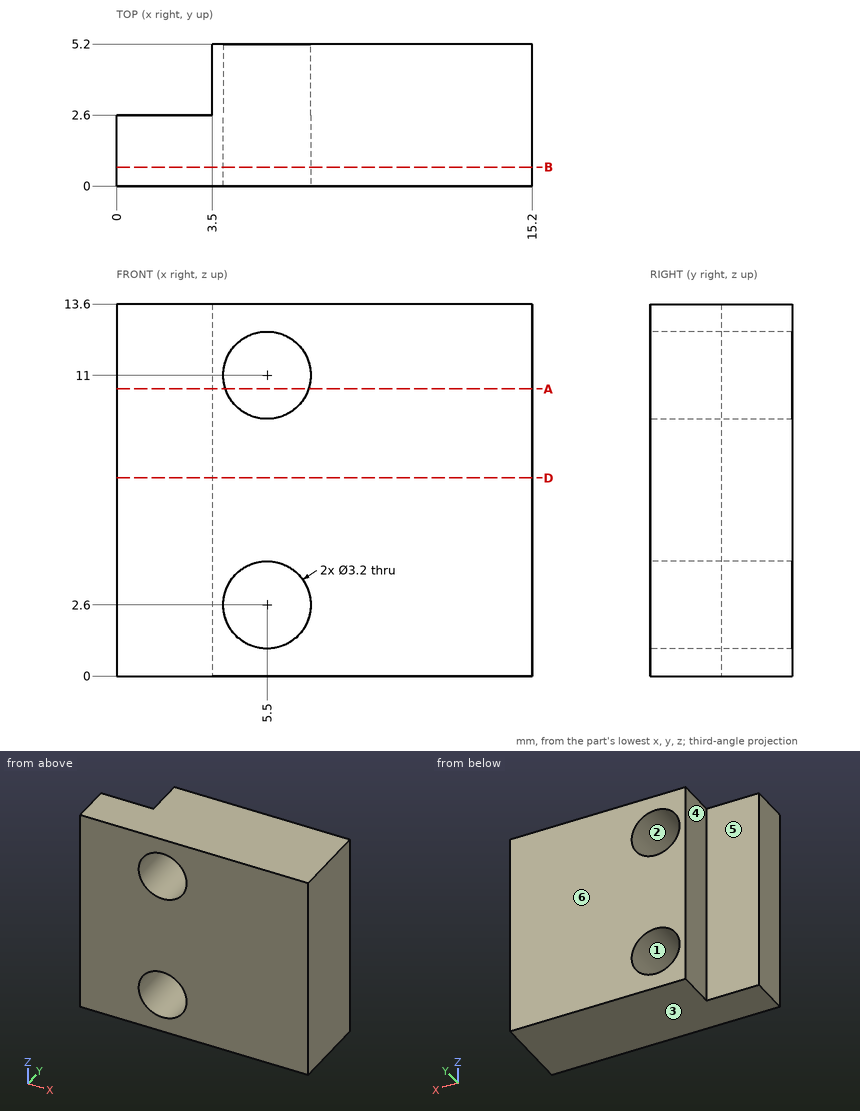
For this review, use the dimensioned drawing (mm, ordinates from the lowest corner) and the shaded views. A direction names the side the tool comes from. Round coordinates to 2 decimals unless told otherwise and drop trailing zeros. Write each loop counter-clockwise with the first axis right and the second up, starting at its lowest first coordinate (ties: lowest second). Pieces come first, ordered by that corner, then holes. Notation, with made-up numbers: (34, 69) - (76, 69) arc R17 cw to (76, 76) - close; hole circle Ø9 at (61, 28). An arc over 180 degrees is marked (long way). Answer as a JSON object with one key per item and string values.
1. Tool access review of the marked faces 5 and 6: name each direction out of +Z, -Z, +X, -X, +Y, -Y from which nothing blocks a thin tool from reaching the whole face with its end or side.
Response values:
{"face 5": "+Z, -Z, -X, +Y", "face 6": "+Z, -Z, +X, -X, +Y"}
2. We need section A-A on z = 10.5. Give the boundary of the cut face in (x, y).
Response values:
{"outline": "(0, 0) - (3.98, 0) - (3.98, 5.2) - (3.5, 5.2) - (3.5, 2.6) - (0, 2.6) - close; (7.02, 0) - (15.2, 0) - (15.2, 5.2) - (7.02, 5.2) - close"}
3. We need section D-D on z = 7.25. Give the boundary of the cut face in (x, y).
Response values:
{"outline": "(0, 0) - (15.2, 0) - (15.2, 5.2) - (3.5, 5.2) - (3.5, 2.6) - (0, 2.6) - close"}
4. For pin 1 Ø3 at (x, z) = (5.5, 11) entering from -Y; pin 2 Ø2 at (y, z) = (4, 8) entering from -X; pin 3 Ø1 at (x, z) = (2, 7) entering from +Y, all flat-tipped, find the tip position at first contact; note any pin that passes through.
Response values:
{"pin 1": "passes through", "pin 2": "stops at x = 3.5", "pin 3": "stops at y = 2.6"}
5. To check wall thickness, follow line 1 along Z through (x, y) = (5.5, 1.3); line 2 along X through (y, z) = (1.7, 2.6); line 3 along X through (y, z) = (2.8, 11). State the ranges of each line that lie inside material, in increasing order.
Response values:
{"line 1": "z = 0 to 1, 4.2 to 9.4, 12.6 to 13.6", "line 2": "x = 0 to 3.9, 7.1 to 15.2", "line 3": "x = 3.5 to 3.9, 7.1 to 15.2"}
6. We need section B-B on y = 0.7. Give the boundary of the cut face in (x, z).
Response values:
{"outline": "(0, 0) - (15.2, 0) - (15.2, 13.6) - (0, 13.6) - close; hole circle Ø3.2 at (5.5, 2.6); hole circle Ø3.2 at (5.5, 11)"}
7. Draft analysis for pull direction Z (two halves, no side actions). For the marked faces 1, 2, 3 and 4, state which applies: +Z half, -Z half, draft (parallel to the pull), parting line (faces both ways), or undercut.
Response values:
{"face 1": "undercut", "face 2": "undercut", "face 3": "-Z half", "face 4": "draft"}
